Read the model definition and answer for the solid it produces. Units are mm, in the model's axes. A direction names the side the tool comes from. Coordinates: 2 decimals unless noted, no trailing zeros. Loops run counter-clockwise (first coordinate to the right, second up) from the corner with the lowest first, then second, coordinate; pieces in that order, holes last. Notation, with made-up numbers: (50, 56.25) - (71, 56.25) arc R4 ccw to (71, 60.25) - close; hole circle Ø11 at (26.5, 17.5). An arc over 180 degrees is marked (long way). Use one line per item in the form item = value. Start each with the question number.
1) A cutting plane is placed at C-C (y = 0.75). State how many separate pieces and enclosed holes the cut face has, and give its area (3 significant figures).
2) A cutting plane is placed at D-D (z = 6.75). Give the vertices of the cut face in (x, y), and give its area (3 significant figures).
3) A cutting plane is placed at B-B (x = 14.5). Give the vertices of the cut face in (y, z).
4) The mould has two halves that part along Y. Classify faces 6 (the face through (14.68, -5.52, 1.25)), 7 (the face through (33.146, -0.09, 1.252)), 8 (the face through (26.545, 0.061, 1.252)), 9 (the face through (13, 0, 2.54)): released by +Y, released by -Y, zero draft, split by the parting line, or undercut.
5) A cutting plane is placed at A-A (z = 1.5). Give the vertices of the cut face in (x, y), and give its area (3 significant figures).
6) Consider line 1 (X direction, y = -1.25, z = 0.75); line 2 (Z direction, x = 11.5, y = 5.75); line 3 (Z direction, x = -1, y = -2). Determine where each line is inside the solid, lowest interval first.
7) Each of these flat-tipped pins is pushed along its axis until it touches: P1, Ø1.8, axis at x = 0, y = 1, coming from the -Z side; P2, Ø4.5, axis at x = 27.94, y = 0, coming from the +Z side; P3, Ø1.5, axis at y = -1, z = 3.5, coming from the +X side. Where does it stop, or does it pass through?
8) Which of the six approach directions +Z, -Z, +X, -X, +Y, -Y give full straight-line access (tool end or side, diameter ignored) to faces 1 (the face through (2.2, -2.2, 7.62)), 2 (the face through (-3, 3, -0.254)), 3 (the face through (-4, 4, 0)), 4 (the face through (-0.661, 5.037, 5.044)), 5 (the face through (-0.633, -2.852, 1.252))?
from build123d import *

# Parameters (mm, degrees)
SKETCH1_R           = 2.921
SKETCH1_R_2         = 1.397
BOSS_EXTRUDE1_DEPTH = 2.54
SKETCH2_R           = 5.08
SKETCH2_R_2         = 2.921
BOSS_EXTRUDE2_DEPTH = 5.08
SKETCH3_R           = 2.921
SKETCH3_R_2         = 1.8415
BOSS_EXTRUDE3_DEPTH = 1.27
BOSS_EXTRUDE4_DEPTH = 0.254


with BuildPart() as part:
    # Sketch1 → Boss-Extrude1 (new body)
    with BuildSketch(Plane.XY):
        with BuildLine():
            ThreePointArc((29.190418502, -4.302847972), (33.147, 0), (29.190418502, 4.302847972))
            Line((29.190418502, 4.302847972), (0.563387665, 6.707380662))
            ThreePointArc((0.563387665, 6.707380662), (-6.731, 0), (0.563387665, -6.707380662))
            Line((0.563387665, -6.707380662), (29.190418502, -4.302847972))
        make_face()
        Circle(SKETCH1_R, mode=Mode.SUBTRACT)
        with Locations((15.466782925, 0)):
            Circle(SKETCH1_R_2, mode=Mode.SUBTRACT)
        with Locations((27.940644271, 0)):
            Circle(SKETCH1_R_2, mode=Mode.SUBTRACT)
    extrude(amount=BOSS_EXTRUDE1_DEPTH)

    # Sketch2 → Boss-Extrude2 (add)
    with BuildSketch(Plane.XY.offset(2.54)):
        Circle(SKETCH2_R)
        Circle(SKETCH2_R_2, mode=Mode.SUBTRACT)
    extrude(amount=BOSS_EXTRUDE2_DEPTH)

    # Sketch3 → Boss-Extrude3 (add)
    with BuildSketch(Plane.XY.offset(2.54)):
        Circle(SKETCH3_R)
        Circle(SKETCH3_R_2, mode=Mode.SUBTRACT)
    extrude(amount=BOSS_EXTRUDE3_DEPTH)

    # Sketch4 → Boss-Extrude4 (add)
    with BuildSketch(Plane(origin=(0, 0, 0), x_dir=(-1, 0, 0), z_dir=(0, 0, -1))):
        Polygon((6.731, 0), (0, 6.731), (-1.116069724, 5.614930276), (5.614930276, -1.116069724), align=None)
    extrude(amount=BOSS_EXTRUDE4_DEPTH)


solid = part.part
Found:
q1.separate_pieces = 4
q1.enclosed_holes = 0
q1.area = 101 mm^2
q2.outline = circle Ø10.16 at (0, 0); hole circle Ø5.84 at (0, 0)
q2.area = 54.3 mm^2
q3.outline = (-5.54, 0) - (-1.01, 0) - (-1.01, 2.54) - (-5.54, 2.54) - close; (1.01, 0) - (5.54, 0) - (5.54, 2.54) - (1.01, 2.54) - close
q4.face_6 = released by -Y
q4.face_7 = split by the parting line
q4.face_8 = undercut
q4.face_9 = zero draft
q5.outline = (0.56, -6.71) - (29.19, -4.3) arc R4.32 ccw to (29.19, 4.3) - (0.56, 6.71) arc R6.73 ccw (long way) to start; hole circle Ø5.84 at (0, 0); hole circle Ø2.79 at (15.47, 0); hole circle Ø2.79 at (27.94, 0)
q5.area = 381 mm^2
q6.line_1 = -6.61 to -2.64, 2.64 to 14.84, 16.09 to 27.32, 28.56 to 32.96
q6.line_2 = 0 to 2.54
q6.line_3 = 2.54 to 3.81
q7.P1 = 2.54
q7.P2 = 2.54
q7.P3 = 5.07
q8.face_1 = +Z, +X, -X, +Y, -Y
q8.face_2 = -Z, +X, -X, +Y, -Y
q8.face_3 = -Z, -X, +Y
q8.face_4 = +Z
q8.face_5 = -Z
